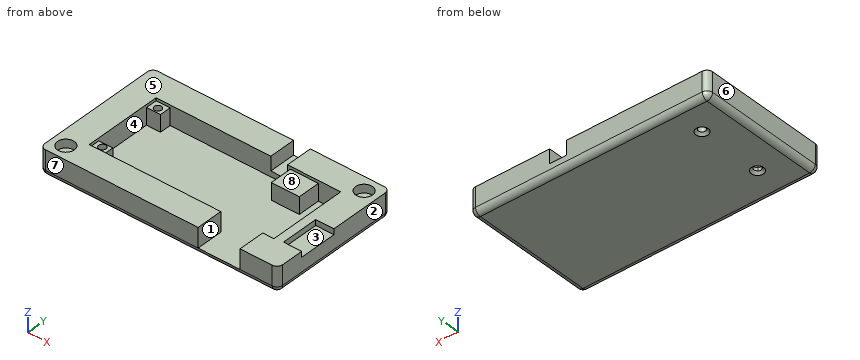
Autodesk Fusion 360 part; units mm, degrees
sketch "Sketch1" plane through (0, 0, 0) normal (0, 0, 1) x (1, 0, 0)
  line L0 (0, 0) -> (65, 0)
  line L1 (65, 0) -> (65, 27)
  line L2 (65, 27) -> (0, 27)
  line L3 (0, 27) -> (0, 0)
  line L4 (-10, -10) -> (75, -10)
  line L5 (75, -10) -> (75, 37)
  line L6 (75, 37) -> (-10, 37)
  line L7 (-10, 37) -> (-10, -10)
  dimension "d3" = 65
  dimension "d4" = 27
  dimension "d5" = 85
  dimension "d6" = 47
  dimension "d7" = 10
  dimension "d8" = 10
extrude "Extrude1" add sketch "Sketch1" along normal blind 2 contours L0 L1 L2 L3 | L4 L5 L6 L7
sketch "Sketch2" plane through (0, 0, 2) normal (0, 0, 1) x (-1, 0, 0)
  line L0 (10, -37) -> (10, 10)
  line L1 (10, 10) -> (-75, 10)
  line L2 (-75, 10) -> (-75, -37)
  line L3 (-75, -37) -> (10, -37)
  line L4 (-65.5, -27.5) -> (0.5, -27.5)
  line L5 (0.5, -27.5) -> (0.5, 0.5)
  line L6 (0.5, 0.5) -> (-65.5, 0.5)
  line L7 (-65.5, 0.5) -> (-65.5, -27.5)
  dimension "d19" = 66
  dimension "d20" = 28
  dimension "d21" = 9.5
  dimension "d22" = 9.5
extrude "Extrude3" add sketch "Sketch2" along normal blind 7
sketch "Sketch3" plane through (0, 0, 2) normal (0, 0, 1) x (-1, 0, 0)
  circle A0 centre (-2.1, -25.25) radius 1.1
  line L0 (0.5, -27.5) -> (0.5, 0.5)
  line L1 (-65.5, -27.5) -> (0.5, -27.5)
  circle A1 centre (-2.1, -1.75) radius 1.1
  line L2 (0.5, 0.5) -> (-65.5, 0.5)
  dimension "d25" = 2.2
  dimension "d26" = 2.6
  dimension "d27" = 2.25
  dimension "d28" = 2.2
  dimension "d29" = 2.25
  dimension "d30" = 2.6
extrude "Extrude4" cut sketch "Sketch3" against normal blind 3
sketch "Sketch4" plane through (0, 0, 9) normal (0, 0, 1) x (-1, 0, 0)
  line L0 (-65.5, -27.5) -> (-65.5, 0.5)
  line L1 (-65.5, 0.5) -> (0.5, 0.5)
  line L2 (0.5, 0.5) -> (0.5, -27.5)
  line L3 (0.5, -27.5) -> (-65.5, -27.5)
  line L4 (-75, -37) -> (10, -37)
  line L5 (10, -37) -> (10, 10)
  line L6 (10, 10) -> (-75, 10)
  line L7 (-75, 10) -> (-75, -37)
  line L8 (-46.5, -37) -> (-40.5, -37)
  line L9 (-40.5, -37) -> (-40.5, -27.5)
  line L10 (-40.5, -27.5) -> (-46.5, -27.5)
  line L11 (-46.5, -27.5) -> (-46.5, -37)
  line L12 (0.5, -27.5) -> (0.5, 0.5)
  line L13 (-65.5, 0.5) -> (-65.5, -27.5)
  dimension "d34" = 41
  dimension "d35" = 19
extrude "Extrude5" cut sketch "Sketch4" against normal blind 5 contours L3 L4 L8 L9 L10 L11
sketch "Sketch7" plane through (0, 0, 9) normal (0, 0, 1) x (-1, 0, 0)
  line L0 (-46.5, -37) -> (-46.5, -27.5)
  line L1 (-46.5, -27.5) -> (-65.5, -27.5)
  line L2 (-65.5, -27.5) -> (-65.5, 0.5)
  line L3 (-65.5, 0.5) -> (0.5, 0.5)
  line L4 (0.5, 0.5) -> (0.5, -27.5)
  line L5 (0.5, -27.5) -> (-40.5, -27.5)
  line L6 (-40.5, -27.5) -> (-40.5, -37)
  line L7 (-40.5, -37) -> (10, -37)
  line L8 (10, -37) -> (10, 10)
  line L9 (10, 10) -> (-75, 10)
  line L10 (-75, 10) -> (-75, -37)
  line L11 (-75, -37) -> (-46.5, -37)
  circle A0 centre (5, 5) radius 3
  circle A1 centre (-70, -32) radius 3
  dimension "d52" = 6
  dimension "d53" = 5
  dimension "d54" = 5
  dimension "d55" = 6
  dimension "d56" = 5
  dimension "d57" = 5
extrude "Extrude7" cut sketch "Sketch7" against normal blind 3 contours A0 | A1
sketch "Sketch8" plane through (0, 0, 9) normal (0, 0, 1) x (-1, 0, 0)
  circle A0 centre (5, 5) radius 3
  circle A1 centre (-70, -32) radius 3
  line L0 (-46.5, -37) -> (-46.5, -27.5)
  line L1 (-46.5, -27.5) -> (-65.5, -27.5)
  line L2 (-65.5, -27.5) -> (-65.5, 0.5)
  line L3 (-65.5, 0.5) -> (0.5, 0.5)
  line L4 (0.5, 0.5) -> (0.5, -27.5)
  line L5 (0.5, -27.5) -> (-40.5, -27.5)
  line L6 (-40.5, -27.5) -> (-40.5, -37)
  line L7 (-40.5, -37) -> (10, -37)
  line L8 (10, -37) -> (10, 10)
  line L9 (10, 10) -> (-75, 10)
  line L10 (-75, 10) -> (-75, -37)
  line L11 (-75, -37) -> (-46.5, -37)
  line L12 (-46.5, 0.5) -> (-61.5, 0.5)
  line L13 (-61.5, 0.5) -> (-61.5, 10)
  line L14 (-61.5, 10) -> (-46.5, 10)
  line L15 (-46.5, 10) -> (-46.5, 0.5)
  line L16 (0.5, -27.5) -> (0.5, 0.5)
  line L17 (-65.5, 0.5) -> (-65.5, -27.5)
  dimension "d61" = 47
  dimension "d62" = 4
extrude "Extrude8" cut sketch "Sketch8" against normal blind 7 contours L3 L9 L12 L13 L14 L15
fillet "Fillet1" radius 2 4 edges at (-10, -10, 4.5) (75, -10, 4.5) (75, 37, 4.5) (-10, 37, 4.5)
sketch "Sketch9" plane through (0, 0, 9) normal (0, 0, 1) x (-1, 0, 0)
  arc A0 (-75, -35) -> (-73, -37) centre (-73, -35) ccw
  line L0 (-73, -37) -> (-46.5, -37)
  line L1 (-46.5, -37) -> (-46.5, -27.5)
  line L2 (-46.5, -27.5) -> (-65.5, -27.5)
  line L3 (-65.5, -27.5) -> (-65.5, 0.5)
  line L4 (-65.5, 0.5) -> (-61.5, 0.5)
  line L5 (-61.5, 0.5) -> (-61.5, 10)
  line L6 (-61.5, 10) -> (-73, 10)
  arc A1 (-73, 10) -> (-75, 8) centre (-73, 8) ccw
  line L7 (-75, 8) -> (-75, -35)
  circle A2 centre (-70, -32) radius 3
  line L8 (-75, 0) -> (-68.5, 0)
  line L9 (-68.5, 0) -> (-68.5, -13.5)
  line L10 (-68.5, -13.5) -> (-75, -13.5)
  line L11 (-75, -13.5) -> (-75, 0)
  line L12 (-65.5, 0.5) -> (-65.5, -27.5)
  dimension "d67" = 10
  dimension "d68" = 3
  dimension "d69" = 13.5
extrude "Extrude9" cut sketch "Sketch9" against normal blind 2 contours L7 L8 L9 L10 L11
sketch "Sketch10" plane through (0, 0, 0) normal (0, 0, -1) x (1, 0, 0)
  arc A0 (-10, -35) -> (-8, -37) centre (-8, -35) ccw
  line L0 (-8, -37) -> (73, -37)
  arc A1 (73, -37) -> (75, -35) centre (73, -35) ccw
  line L1 (75, -35) -> (75, 8)
  arc A2 (75, 8) -> (73, 10) centre (73, 8) ccw
  line L2 (73, 10) -> (-8, 10)
  arc A3 (-8, 10) -> (-10, 8) centre (-8, 8) ccw
  line L3 (-10, 8) -> (-10, -35)
  circle A4 centre (2.1, -25.25) radius 1.1
  circle A5 centre (2.1, -1.75) radius 1.1
  line L4 (-0.5, 0.5) -> (65.5, 0.5)
  line L5 (-0.5, -27.5) -> (-0.5, 0.5)
  circle A6 centre (2.1, -25.25) radius 1.1
  circle A7 centre (2.1, -1.75) radius 1.1
  dimension "d75" = 2.2
hole "Hole1" at (2.1, 2, 0) at (2.1, 25.25, 0) direction (0, 0, 1) diameter 2.6 depth 14 tip angle 180 countersink diameter 4.4 countersink angle 90
sketch "Sketch11" plane through (0, 0, 2) normal (0, 0, 1) x (-1, 0, 0)
  line L0 (-65.5, -27.5) -> (0.5, -27.5)
  line L1 (0.5, -27.5) -> (0.5, 0.5)
  line L2 (0.5, 0.5) -> (-46.5, 0.5)
  line L3 (-46.5, 0.5) -> (-46.5, 10)
  line L4 (-46.5, 10) -> (-61.5, 10)
  line L5 (-61.5, 10) -> (-61.5, 0.5)
  line L6 (-61.5, 0.5) -> (-65.5, 0.5)
  line L7 (-65.5, 0.5) -> (-65.5, -27.5)
  arc A0 (-2.8161, -0.915) -> (-1.3839, -0.915) centre (-2.1, -2) ccw
  arc A1 (-1.3839, -0.915) -> (-2.8161, -0.915) centre (-2.1, -1.75) ccw
  circle A2 centre (-2.1, -25.25) radius 1.3
  line L8 (0.5, -27.5) -> (-4.5, -27.5)
  line L9 (-4.5, -27.5) -> (-4.5, -23.5)
  line L10 (-4.5, -23.5) -> (0.5, -23.5)
  line L11 (0.5, -23.5) -> (0.5, -27.5)
  line L12 (0.5, 0.5) -> (-4.5, 0.5)
  line L13 (-4.5, 0.5) -> (-4.5, -3.5)
  line L14 (-4.5, -3.5) -> (0.5, -3.5)
  line L15 (0.5, -3.5) -> (0.5, 0.5)
  dimension "d81" = 5
  dimension "d82" = 4
  dimension "d83" = 5
  dimension "d84" = 4
extrude "Extrude10" add sketch "Sketch11" along normal blind 6 contours L0 L1 L8 L9 L10 L11 | L1 L2 L12 L13 L14 L15
sketch "Sketch12" plane through (0, 0, 2) normal (0, 0, 1) x (-1, 0, 0)
  line L0 (-4.5, -27.5) -> (-4.5, -23.5)
  line L1 (-4.5, -23.5) -> (0.5, -23.5)
  line L2 (0.5, -23.5) -> (0.5, -3.5)
  line L3 (0.5, -3.5) -> (-4.5, -3.5)
  line L4 (-4.5, -3.5) -> (-4.5, 0.5)
  line L5 (-4.5, 0.5) -> (-46.5, 0.5)
  line L6 (-46.5, 0.5) -> (-46.5, 10)
  line L7 (-46.5, 10) -> (-61.5, 10)
  line L8 (-61.5, 10) -> (-61.5, 0.5)
  line L9 (-61.5, 0.5) -> (-65.5, 0.5)
  line L10 (-65.5, 0.5) -> (-65.5, -27.5)
  line L11 (-65.5, -27.5) -> (-4.5, -27.5)
  line L12 (-47.5, -27.5) -> (-57.5, -27.5)
  line L13 (-57.5, -27.5) -> (-57.5, -19.5)
  line L14 (-57.5, -19.5) -> (-47.5, -19.5)
  line L15 (-47.5, -19.5) -> (-47.5, -27.5)
  dimension "d87" = 10
  dimension "d88" = 8
  dimension "d89" = 18
extrude "Extrude11" add sketch "Sketch12" along normal blind 6 contours L11 L12 L13 L14 L15
fillet "Fillet2" radius 2 8 edges at (75, 13.5, 0) (74.4142, 36.4142, 0) (32.5, 37, 0) (-9.4142, 36.4142, 0) (-10, 13.5, 0) (-9.4142, -9.4142, 0) (32.5, -10, 0) (74.4142, -9.4142, 0)
Check sheet for the modelled part. Datum: model origin and axes. Units: mm. Face numbers are marked on the shaded views. A direction names the side the tool comes from. Round coordinates to 2 decimals unless told otherwise and drop trailing zeros. Loops run counter-clockwise (first coordinate to the right, second up) from the corner with the lowest first, then second, coordinate; pieces in that order, holes last. Notation, with made-up numbers: M 68,73 L 78,73 A10 ccw 78,79 Z; hole C 56,-17.75 d5. An arc over 180 degrees is marked long. One line per question, with ' | ' between items. Start each with the question number.
Item 1: Gauge pin test, flat ends, axial feed: pin 1 Ø19 at (x, y) = (37.5, 12.5) entering from +Z; pin 2 Ø1.8 at (x, y) = (42.5, 32) entering from +Z; pin 3 Ø1.8 at (x, y) = (-5, -5) entering from +Z. Record the tip position at first contact, or that the pin passes through.
Item 2: Release check for a two-part mould opening along X. For the marked faces 6, 7 and 8 record: released by +X, released by -X, zero draft, split by the parting line, or undercut.
Item 3: Section check B-B (x = 70). Record the boundary of the cut face in (y, z), and give its area (3 significant figures).
Item 4: Scan lines: probe 1 along X at (y, z) = (-5, 7.15); probe 2 along Y at (x, z) = (14.5, 8); probe 3 along Y at (x, z) = (2.1, 6.25). Record each from-to range of solid material in increasing order.
Item 5: Section check D-D (y = 16). Record the boundary of the cut face in (x, z), and give its area (3 significant figures).
Item 6: Set-up check for the marked faces 1, 2, 3, 4 and 5: record each of +Z, -Z, +X, -X, +Y, -Y from which the full face is reachable in a straight line by a thin tool's end or side.
Item 7: Section check C-C (z = 3). Record the boundary of the cut face in (x, y) (3 decimals).
Item 8: Section check A-A (y = 25.25). Record the boundary of the cut face in (x, z), and give its area (3 significant figures).
Worked out:
1) pin 1: z = 2 | pin 2: z = 4 | pin 3: z = 6
2) face 6: released by -X | face 7: zero draft | face 8: undercut
3) outline: M -10,2 A2 ccw -8,0 L 35,0 A2 ccw 37,2 L 37,9 L 35,9 L 35,6 L 29,6 L 29,9 L 13.5,9 L 13.5,7 L 0,7 L 0,9 L -10,9 Z | area: 376 mm^2
4) probe 1: -10 to -8, -2 to 46.5, 61.5 to 75 | probe 2: -10 to -0.5, 27.5 to 37 | probe 3: -10 to 0.65, 3.3 to 3.5, 23.5 to 23.95, 26.55 to 37
5) outline: M -10,2 A2 ccw -8,0 L 73,0 A2 ccw 75,2 L 75,9 L 65.5,9 L 65.5,2 L -0.5,2 L -0.5,9 L -10,9 Z | area: 301 mm^2
6) face 1: +Z, -Y | face 2: +Z, -Z, +X, +Y, -Y | face 3: +Z, +X | face 4: +Z | face 5: +Z, +X, -X, +Y, -Y
7) outline: M -10,-8 A2 ccw -8,-10 L 46.5,-10 L 46.5,-0.5 L 4.5,-0.5 L 4.5,3.5 L -0.5,3.5 L -0.5,23.5 L 4.5,23.5 L 4.5,27.5 L 47.5,27.5 L 47.5,19.5 L 57.5,19.5 L 57.5,27.5 L 65.5,27.5 L 65.5,-0.5 L 61.5,-0.5 L 61.5,-10 L 73,-10 A2 ccw 75,-8 L 75,35 A2 ccw 73,37 L -8,37 A2 ccw -10,35 Z; hole C 2.1,25.25 d2.6; hole M 1.384,0.915 A1.1 ccw 2.816,0.915 A1.3 ccw long Z
8) outline: M -10,2 A2 ccw -8,0 L -0.1,0 L 0.8,0.9 L 0.8,8 L -0.5,8 L -0.5,9 L -10,9 Z; M 3.4,0.9 L 4.3,0 L 73,0 A2 ccw 75,2 L 75,9 L 65.5,9 L 65.5,2 L 57.5,2 L 57.5,8 L 47.5,8 L 47.5,2 L 4.5,2 L 4.5,8 L 3.4,8 Z | area: 370 mm^2
